CAD build for the part. Positions are in the model's coordinates, mm. Face numbers are marked on the shaded views. A direction names the side the tool comes from. Round coordinates to 2 decimals unless told otherwise and drop trailing zeros. Write each loop counter-clockwise with the first axis right and the second up, starting at its lowest first coordinate (ties: lowest second). Pieces come first, ordered by that corner, then holes. Notation, with made-up numbers: (-27, -18) - (-17, -18) arc R9 ccw to (-17, -13) - close; hole circle Ø8 at (8.25, -20.5). An arc over 180 degrees is marked (long way). Put each result on its own line as item: value. Start each with the question number.
Item 1: Pin check, flat tips, straight feed: pin 1 Ø4 at (x, z) = (-6.92, 0) entering from +Y; pin 2 Ø2.5 at (x, z) = (6.92, 0) entering from -Y; pin 3 Ø4 at (x, z) = (-1.5, 0) entering from -Y; pin 4 Ø1 at (x, y) = (-4.5, -6) entering from +Z. Stop position of each tip, or through.
Item 2: Cut at C-C (x = 7.5). Give the cut face in (y, z).
Item 3: Cut at A-A (x = 0). Give the cut face in (y, z).
Item 4: Mould opens along X. For the marked faces 1, 2 and 3 say: released by +X, released by -X, zero draft, split by the parting line, or undercut.
Item 5: Cut at B-B (z = 0). Give the cut face in (x, y).
Item 6: 3-axis set-ups, long thin cutter, end or side, ignore diameter. For the marked faces 4 and 5: which of +Z, -Z, +X, -X, +Y, -Y reach the whole face in a straight line?
Item 7: Cut at D-D (y = -4.75). Count the separate pieces of the cut face and the enclosed holes in it, and give its area (3 significant figures).
Item 8: Drill centre lines: line 1 (Z direction, x = 0, y = -12); line 2 (X direction, y = -0.75, z = -4); line 3 (Y direction, x = -4, z = -3.5). Where is each one in solid material? Low to high. Write a range as from..to.
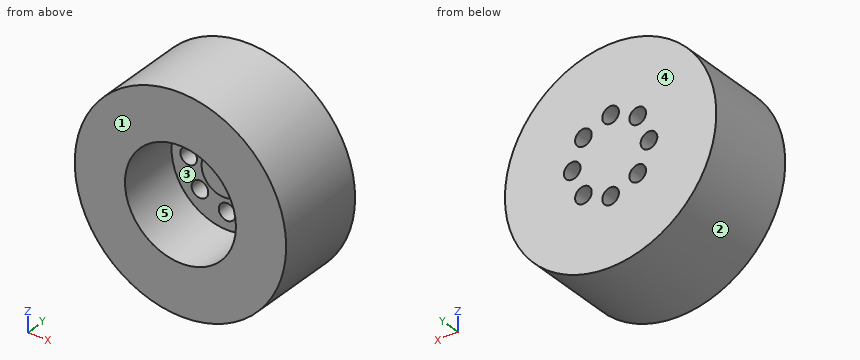
```python
from build123d import *

# Parameters (mm, degrees)
F0_R     = 19.05
F1_DEPTH = 16.5608
F2_R     = 10
F3_DEPTH = 11.2
F4_R     = 4
F5_DEPTH = 0.8
F8_R     = 1.5
F9_DEPTH = 6


# Not quite as in the source:
# - the program builds the solid bodies; features that only make, move or delete a surface that nothing else refers to are left out


with BuildPart() as f1:
    # F0 (on Front) → F1 (new body)
    with BuildSketch(Plane.XZ):
        Circle(F0_R)
    extrude(amount=F1_DEPTH)

    # F2 (on face) → F3 (cut)
    with BuildSketch(Plane.XZ.offset(16.5608)):
        Circle(F2_R)
    extrude(amount=-F3_DEPTH, mode=Mode.SUBTRACT)

    # F4 (on face) → F5 (join)
    with BuildSketch(Plane.XZ.offset(5.3608)):
        Circle(F4_R)
    extrude(amount=F5_DEPTH)

    # F8 (on face) → F9 (cut)
    with BuildSketch(Plane.XZ.offset(5.3608)):
        with Locations((0, 6.9199060356)):
            Circle(F8_R)
        with Locations((-4.8931124829, 4.8931124829)):
            Circle(F8_R)
        with Locations((-6.9199060356, 0)):
            Circle(F8_R)
        with Locations((-4.8931124829, -4.8931124829)):
            Circle(F8_R)
        with Locations((0, -6.9199060356)):
            Circle(F8_R)
        with Locations((4.8931124829, -4.8931124829)):
            Circle(F8_R)
        with Locations((6.9199060356, 0)):
            Circle(F8_R)
        with Locations((4.8931124829, 4.8931124829)):
            Circle(F8_R)
    extrude(amount=-F9_DEPTH, mode=Mode.SUBTRACT)


solid = f1.part
```
Output values:
1. pin 1: y = 0
1. pin 2: through
1. pin 3: y = -6.16
1. pin 4: z = 18.63
2. outline: (-16.56, -17.51) - (0, -17.51) - (0, -1.38) - (-5.36, -1.38) - (-5.36, -6.61) - (-16.56, -6.61) - close; (-16.56, 6.61) - (-5.36, 6.61) - (-5.36, 1.38) - (0, 1.38) - (0, 17.51) - (-16.56, 17.51) - close
3. outline: (-16.56, -19.05) - (0, -19.05) - (0, -8.42) - (-5.36, -8.42) - (-5.36, -10) - (-16.56, -10) - close; (-16.56, 10) - (-5.36, 10) - (-5.36, 8.42) - (0, 8.42) - (0, 19.05) - (-16.56, 19.05) - close; (-6.16, -4) - (-5.36, -4) - (-5.36, -5.42) - (0, -5.42) - (0, 5.42) - (-5.36, 5.42) - (-5.36, 4) - (-6.16, 4) - close
4. face 1: zero draft
4. face 2: split by the parting line
4. face 3: undercut
5. outline: (-19.05, -16.56) - (-10, -16.56) - (-10, -5.36) - (-8.42, -5.36) - (-8.42, 0) - (-19.05, 0) - close; (-5.42, -5.36) - (-4, -5.36) - (-4, -6.16) - (4, -6.16) - (4, -5.36) - (5.42, -5.36) - (5.42, 0) - (-5.42, 0) - close; (8.42, -5.36) - (10, -5.36) - (10, -16.56) - (19.05, -16.56) - (19.05, 0) - (8.42, 0) - close
6. face 4: +Z, -Z, +X, -X, +Y
6. face 5: -Y
7. separate pieces: 1
7. enclosed holes: 8
7. area: 1,080 mm2
8. line 1: -19.05..-10, 10..19.05
8. line 2: -18.63..-6.1, -3.69..3.69, 6.1..18.63
8. line 3: -5.36..0
